CAD build for the part. Positions are in the model's coordinates, mm. Coordinates: 2 decimals unless noted, no trailing zeros. Loops run counter-clockwise (first coordinate to the right, second up) from the corner with the lowest first, then second, coordinate; pieces in that order, holes last. Notation, with made-up numbers: (4, -0.5) -> (34, -0.5) arc R7 ccw to (34, 9.5) -> close; hole circle Ø6 at (-36.5, 6.5). An arc over 180 degrees is marked (long way). Write each question's results on one line, items separated by ' | '.
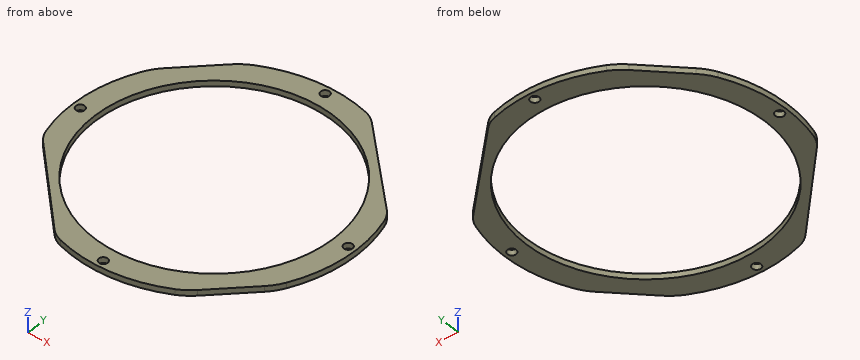
from build123d import *

# Parameters (mm, degrees)
SKETCH_1_R          = 50.45
SKETCH_1_R_2        = 1.55
SKETCH_1_R_3        = 42.5
EXTRUDE_1_DEPTH     = 2
CUT_EXTRUDE_START   = -8
CUT_EXTRUDE_1_DEPTH = 8
FILLET_1_R          = 20
CUT_EXTRUDE_2_DEPTH = 10
CUT_EXTRUDE_3_DEPTH = 10
FILLET_2_R          = 10


with BuildPart() as part:
    # 草图1 → 凸台-拉伸1 (new body)
    with BuildSketch(Plane.XY):
        Circle(SKETCH_1_R)
        with Locations((0, 47.7)):
            Circle(SKETCH_1_R_2, mode=Mode.SUBTRACT)
        with Locations((47.7, 0)):
            Circle(SKETCH_1_R_2, mode=Mode.SUBTRACT)
        with Locations((0, -47.7)):
            Circle(SKETCH_1_R_2, mode=Mode.SUBTRACT)
        with Locations((-47.7, 0)):
            Circle(SKETCH_1_R_2, mode=Mode.SUBTRACT)
        Circle(SKETCH_1_R_3, mode=Mode.SUBTRACT)
    extrude(amount=EXTRUDE_1_DEPTH)

    # 草图2 → 切除-拉伸1 (cut)
    with BuildSketch(Plane.XY.offset(2).offset(CUT_EXTRUDE_START)):
        with BuildLine():
            Line((-26.156986786, 43.13947777), (-43.13947777, 26.156986786))
            ThreePointArc((-43.13947777, 26.156986786), (-35.673537111, 35.673537111), (-26.156986786, 43.13947777))
        make_face()
        with BuildLine():
            Line((43.13947777, 26.156986786), (26.156986786, 43.13947777))
            ThreePointArc((26.156986786, 43.13947777), (35.673537111, 35.673537111), (43.13947777, 26.156986786))
        make_face()
        with BuildLine():
            Line((26.156986786, -43.13947777), (43.13947777, -26.156986786))
            ThreePointArc((43.13947777, -26.156986786), (35.673537111, -35.673537111), (26.156986786, -43.13947777))
        make_face()
        with BuildLine():
            Line((-43.13947777, -26.156986786), (-26.156986786, -43.13947777))
            ThreePointArc((-26.156986786, -43.13947777), (-35.673537111, -35.673537111), (-43.13947777, -26.156986786))
        make_face()
    extrude(amount=CUT_EXTRUDE_1_DEPTH, mode=Mode.SUBTRACT)

    # 圆角1
    fillet_1_edges = [part.edges().sort_by_distance(p)[0] for p in [
        (-26.156986786, 43.13947777, 1),
        (-43.13947777, 26.156986786, 1),
        (43.13947777, 26.156986786, 1),
        (26.156986786, 43.13947777, 1),
        (26.156986786, -43.13947777, 1),
        (43.13947777, -26.156986786, 1),
        (-43.13947777, -26.156986786, 1),
        (-26.156986786, -43.13947777, 1),
    ]]
    fillet(fillet_1_edges, radius=FILLET_1_R)

    # 草图4 → 切除-拉伸2 (cut)
    with BuildSketch(Plane.XY.offset(2)):
        Polygon((-18.704164587, -51.054840678), (-51.986667617, -16.922686111), (-49.480801159, -14.479198174), (-16.19829813, -48.611352741), align=None)
        Polygon((48.611352741, 16.19829813), (51.054840678, 18.704164587), (16.922686111, 51.986667617), (14.479198174, 49.480801159), align=None)
    extrude(amount=-CUT_EXTRUDE_2_DEPTH, mode=Mode.SUBTRACT)


with BuildPart() as cut_extrude_2_piece_1:
    # of the separate pieces the step leaves, piece 1, a body of its own (cut_extrude_2_pieces)
    add(part.part.solids().sort_by_distance((44.852039635, -23.097554862, 0))[0])

    # 圆角2
    fillet_2_edges = [cut_extrude_2_piece_1.edges().sort_by_distance(p)[0] for p in [
        (-17.437312859, -47.340707855, 1),
        (47.340707855, 17.437312859, 1),
        (16.238659163, 47.765138423, 1),
        (-47.765138423, -16.238659163, 1),
    ]]
    fillet(fillet_2_edges, radius=FILLET_2_R)


with BuildPart() as cut_extrude_2_piece_2:
    # of the separate pieces the step leaves, piece 2, a body of its own (cut_extrude_2_pieces)
    add(part.part.solids().sort_by_distance((-36.822783654, -32.473680902, 0))[0])


with BuildPart() as cut_extrude_2_piece_3:
    # of the separate pieces the step leaves, piece 3, a body of its own (cut_extrude_2_pieces)
    add(part.part.solids().sort_by_distance((32.473680902, 36.822783654, 0))[0])


with BuildPart() as cut_extrude_3_tool:
    # 草图5 → 切除-拉伸3 (new body)
    with BuildSketch(Plane.XY.offset(2)):
        with BuildLine():
            Line((-36.822783654, -32.473680902), (-42.579696276, -26.569803082))
            ThreePointArc((-42.579696276, -26.569803082), (-41.915837064, -27.343862298), (-41.213386503, -28.083078053))
            Line((-41.213386503, -28.083078053), (-36.822783654, -32.473680902))
        make_face()
        with BuildLine():
            Line((26.569803082, 42.579696276), (32.473680902, 36.822783654))
            Line((32.473680902, 36.822783654), (28.083078053, 41.213386503))
            ThreePointArc((28.083078053, 41.213386503), (27.343862298, 41.915837064), (26.569803082, 42.579696276))
        make_face()
    extrude(amount=-CUT_EXTRUDE_3_DEPTH)


with BuildPart() as cut_extrude_2_piece_2_1:
    add(cut_extrude_2_piece_2.part)

    # 切除-拉伸3: cut by cut_extrude_3_tool
    add(cut_extrude_3_tool.part, mode=Mode.SUBTRACT)


with BuildPart() as cut_extrude_2_piece_3_1:
    add(cut_extrude_2_piece_3.part)

    # 切除-拉伸3: cut by cut_extrude_3_tool
    add(cut_extrude_3_tool.part, mode=Mode.SUBTRACT)


solid = cut_extrude_2_piece_1.part
1) Pin check, flat tip, straight feed: pin 1 (3 mm diameter, centred on x = 0, y = 47.7, fed in from +Z). Stop position of the tip, or through.
Outcome:
pin 1: passes through
2) Drill centre lines: L1, parallel to Y at x = 0, z = 0.85; L2, parallel to X at y = -0.5, z = 1.85; L3, parallel to Y at x = 1, z = 0.9. Where is each one in solid material? Low to high. Write a range as from..to.
Outcome:
L1: y = -50.45..-49.25, -46.15..-42.5, 42.5..46.15, 49.25..50.45 | L2: x = -50.45..-49.17, -46.23..-42.5, 42.5..46.23, 49.17..50.45 | L3: y = -50.44..-48.88, -46.52..-42.49, 42.49..46.52, 48.88..50.44
3) Slice it at A-A (x = 0). Write the cut outline in (y, z).
Outcome:
outline: (-50.45, 0) -> (-49.25, 0) -> (-49.25, 2) -> (-50.45, 2) -> close; (-46.15, 0) -> (-42.5, 0) -> (-42.5, 2) -> (-46.15, 2) -> close; (42.5, 0) -> (46.15, 0) -> (46.15, 2) -> (42.5, 2) -> close; (49.25, 0) -> (50.45, 0) -> (50.45, 2) -> (49.25, 2) -> close
4) Slice it at B-B (z = 0.9). Write the cut outline in (x, y), then the cut area to 3 significant figures.
Outcome:
outline: (-48.56, -13.68) arc R10 ccw to (-46.09, -17.95) -> (-19.11, -45.63) arc R10 ccw to (-14.9, -48.2) arc R50.45 ccw to (23.1, -44.85) arc R20 ccw to (28.08, -41.21) -> (41.21, -28.08) arc R20 ccw to (44.85, -23.1) arc R50.45 ccw to (48.2, 14.9) arc R10 ccw to (45.63, 19.11) -> (17.95, 46.09) arc R10 ccw to (13.68, 48.56) arc R50.45 ccw to (-23.1, 44.85) arc R20 ccw to (-28.08, 41.21) -> (-41.21, 28.08) arc R20 ccw to (-44.85, 23.1) arc R50.45 ccw to start; hole circle Ø3.1 at (-47.7, 0); hole circle Ø85 at (0, 0); hole circle Ø3.1 at (0, -47.7); hole circle Ø3.1 at (0, 47.7); hole circle Ø3.1 at (47.7, 0) | area: 1,950 mm^2
5) Slice it at D-D (x = -35). Write the cut outline in (y, z), then the cut area to 3 significant figures.
Outcome:
outline: (-29.33, 0) -> (-24.11, 0) -> (-24.11, 2) -> (-29.33, 2) -> close; (24.11, 0) -> (34.3, 0) -> (34.3, 2) -> (24.11, 2) -> close | area: 30.8 mm^2
